from build123d import *

# Parameters (mm, degrees)
SKETCH1_W           = 114.3
SKETCH1_H           = 177.8
SKETCH1_W_2         = 101.6
SKETCH1_H_2         = 165.1
BOSS_EXTRUDE1_DEPTH = 4.7625
SKETCH2_W           = 12.38677804
SKETCH2_H           = 4.7625
SKETCH2_W_2         = 12.7
BOSS_EXTRUDE2_DEPTH = 4.7625
SKETCH3_W           = 12.7
SKETCH3_H           = 4.7625
BOSS_EXTRUDE3_DEPTH = 4.7625
FILLET1_R           = 2.54


with BuildPart() as part:
    # Sketch1 → Boss-Extrude1 (new body)
    with BuildSketch(Plane(origin=(0, 0, 0), x_dir=(1, 0, 0), z_dir=(0, 1, 0))):
        Rectangle(SKETCH1_W, SKETCH1_H)
        Rectangle(SKETCH1_W_2, SKETCH1_H_2, mode=Mode.SUBTRACT)
    extrude(amount=BOSS_EXTRUDE1_DEPTH)

    # Sketch2 → Boss-Extrude2 (add)
    with BuildSketch(Plane.XY.offset(88.9)):
        with Locations((-38.1, 2.38125)):
            Rectangle(SKETCH2_W, SKETCH2_H)
        with Locations((12.7, 2.38125)):
            Rectangle(SKETCH2_W_2, SKETCH2_H)
    extrude(amount=BOSS_EXTRUDE2_DEPTH)

    # Sketch3 → Boss-Extrude3 (add)
    with BuildSketch(Plane(origin=(0, 0, -88.9), x_dir=(-1, 0, 0), z_dir=(0, 0, -1))):
        with Locations((-38.1, 2.38125)):
            Rectangle(SKETCH3_W, SKETCH3_H)
        with Locations((12.7, 2.38125)):
            Rectangle(SKETCH3_W, SKETCH3_H)
    extrude(amount=BOSS_EXTRUDE3_DEPTH)

    # Fillet1
    fillet1_edges = [part.edges().sort_by_distance(p)[0] for p in [
        (50.8, 2.38125, 82.55),
        (50.8, 2.38125, -82.55),
        (-50.8, 2.38125, -82.55),
        (-50.8, 2.38125, 82.55),
    ]]
    fillet(fillet1_edges, radius=FILLET1_R)


solid = part.part
Part model, mm, in its own coordinate system. A direction names the side the tool comes from. Round coordinates to 2 decimals unless told otherwise and drop trailing zeros. Write each loop counter-clockwise with the first axis right and the second up, starting at its lowest first coordinate (ties: lowest second). Pieces come first, ordered by that corner, then holes. Notation, with made-up numbers: (74.25, -16) - (117.25, -16) arc R12 cw to (117.25, -8) - close; hole circle Ø2 at (15, 0). An arc over 180 degrees is marked (long way). Use CSV: the item, a comma, the result in double quotes.
Item 1: Slice it at B-B, the plane x = 29.5. Write the cut outline in (y, z), then the cut area to 3 significant figures.
Results list:
outline,"(0, -88.9) - (4.76, -88.9) - (4.76, -82.55) - (0, -82.55) - close; (0, 82.55) - (4.76, 82.55) - (4.76, 88.9) - (0, 88.9) - close"
area,"60.5 mm²"
Item 2: Wall check: L1, parallel to X at y = 1.9, z = -14; L2, parallel to Z at x = 3, y = 4.2; L3, parallel to Z at x = 35.5, y = 3.7. Give the ranges that are in metal, low to high.
Results list:
L1,"x = -57.15 to -50.8, 50.8 to 57.15"
L2,"z = -88.9 to -82.55, 82.55 to 88.9"
L3,"z = -93.66 to -82.55, 82.55 to 88.9"
Item 3: Slice it at A-A, the plane z = -65.5. Write the cut outline in (x, y).
Results list:
outline,"(-57.15, 0) - (-50.8, 0) - (-50.8, 4.76) - (-57.15, 4.76) - close; (50.8, 0) - (57.15, 0) - (57.15, 4.76) - (50.8, 4.76) - close"
Item 4: Slice it at C-C, the plane y = 1.55. Write the cut outline in (x, z).
Results list:
outline,"(-57.15, -88.9) - (-19.05, -88.9) - (-19.05, -93.66) - (-6.35, -93.66) - (-6.35, -88.9) - (31.75, -88.9) - (31.75, -93.66) - (44.45, -93.66) - (44.45, -88.9) - (57.15, -88.9) - (57.15, 88.9) - (19.05, 88.9) - (19.05, 93.66) - (6.35, 93.66) - (6.35, 88.9) - (-31.91, 88.9) - (-31.91, 93.66) - (-44.29, 93.66) - (-44.29, 88.9) - (-57.15, 88.9) - close; hole (-50.8, -80.01) arc R2.54 ccw to (-48.26, -82.55) - (48.26, -82.55) arc R2.54 ccw to (50.8, -80.01) - (50.8, 80.01) arc R2.54 ccw to (48.26, 82.55) - (-48.26, 82.55) arc R2.54 ccw to (-50.8, 80.01) - close"
Item 5: Tool access for faces 1 (the flat face through (38, 2, 88.9)), 2 (the flat face through (31.75, 2, -91)), 3 (the flat face through (44.45, 2, -91)), 4 (the flat face through (-38, 2, -88.9)): list every direction of +Z, -Z, +X, -X, +Y, -Y with a clear straight run to the whole face (end or side of a thin tool).
Results list:
face 1,"+Z, +X, +Y, -Y"
face 2,"-Z, +Y, -Y"
face 3,"-Z, +X, +Y, -Y"
face 4,"-Z, -X, +Y, -Y"
Item 6: Flat gauge pins, fed straight in: P1, Ø1.4, axis at x = -5, y = 2.5, coming from the -Z side; P2, Ø1.4, axis at y = 3, z = -92.5, coming from the -X side; P3, Ø2.5, axis at x = -9.5, y = 3, coming from the +Z side. Where does each tip first touch, or does it go through?
Results list:
P1,"stops at z = -88.9"
P2,"stops at x = -19.05"
P3,"stops at z = 88.9"
Item 7: Pull direction Z, two halves, no side cores. Call faces 5 (the flat face through (50.8, 2, 1)), 6 (the flat face through (51, 2, -88.9)), 7 (the flat face through (57.15, 2, 1)): pulls with the +Z half, pulls with the -Z half, needs draft (parallel to the pull), parting line crosses it, or undercut.
Results list:
face 5,"undercut"
face 6,"pulls with the -Z half"
face 7,"needs draft"
